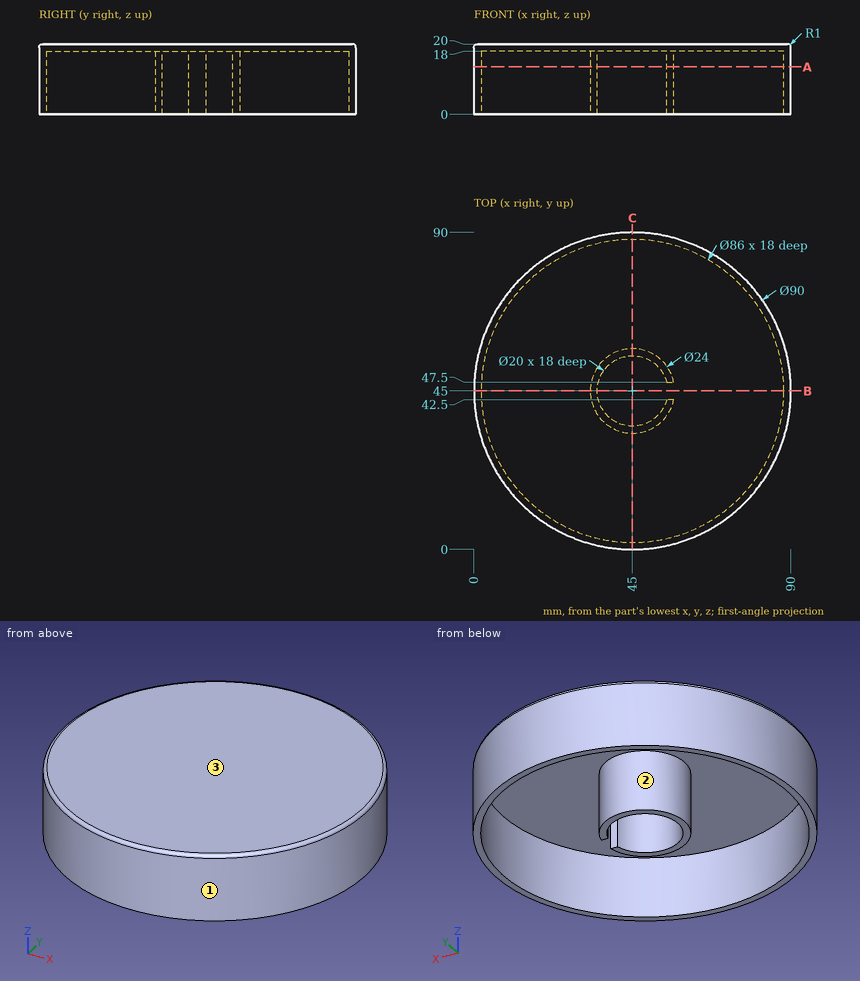
Here's the drawing with two shaded views (mm, measured from the low corner). I have some questions. Coordinates: 2 decimals unless noted, no trailing zeros. Loops run counter-clockwise (first coordinate to the right, second up) from the corner with the lowest first, then second, coordinate; pieces in that order, holes last. Notation, with made-up numbers: M 17,48 L 38,48 A15 ccw 38,58 Z; hole C 7,36.25 d5. An arc over 180 degrees is marked long. Return JSON: item names as keys, results as strings. Group by question number.
Item 1: I'm going to push flat-ended pins straight in: pin 1 Ø5 at (x, z) = (30, 8.5) entering from +Y; pin 2 Ø2.5 at (x, z) = (56, 4.5) entering from +Y; pin 3 Ø0.6 at (x, z) = (55.5, 5) entering from -Y. Where does each tip first touch, or does it pass through?
Item 2: Thinking about a two-plate mould opening in X: for the marked faces 1, 2 and 3, which applies, released by +X, released by -X, zero draft, split by the parting line, or undercut?
Item 3: Imagine slicing it at B-B (y = 45). Please give me the cut outline in (x, z), and give its area (3 significant figures).
Item 4: If I drill on L1, parallel to Y at x = 45, z = 12.75; L2, parallel to X at y = 45.5, z = 17.25; L3, parallel to X at y = 50.5, z = 6.5, over which ranges is the centre line in solid material (lowest first)? Write a range as from..to.
Item 5: Imagine slicing it at A-A (z = 13.5). Please give me the cut outline in (x, y), and give its area (3 significant figures).
Item 6: Imagine slicing it at C-C (x = 45). Please give me the cut outline in (y, z), and give its area (3 significant figures).
Verdict:
{
 "1": {"pin 1": "stops at y = 88.23", "pin 2": "stops at y = 88.93", "pin 3": "stops at y = 1.17"},
 "2": {"face 1": "split by the parting line", "face 2": "undercut", "face 3": "zero draft"},
 "3": {"outline": "M 0,0 L 2,0 L 2,18 L 33,18 L 33,0 L 35,0 L 35,18 L 88,18 L 88,0 L 90,0 L 90,19 A1 ccw 89,20 L 1,20 A1 ccw 0,19 Z", "area": "288 mm^2"},
 "4": {"L1": "y = 0..2, 33..35, 55..57, 88..90", "L2": "x = 0..2, 33.01..35.01, 88..90", "L3": "x = 0.34..2.35, 34.33..36.65, 53.35..55.67, 87.65..89.66"},
 "5": {"outline": "C 45,45 d90; M 54.68,42.5 A10 cw long 54.68,47.5 L 56.74,47.5 A12 ccw long 56.74,42.5 Z; hole C 45,45 d86", "area": "681 mm^2"},
 "6": {"outline": "M 0,0 L 2,0 L 2,18 L 33,18 L 33,0 L 35,0 L 35,18 L 55,18 L 55,0 L 57,0 L 57,18 L 88,18 L 88,0 L 90,0 L 90,19 A1 ccw 89,20 L 1,20 A1 ccw 0,19 Z", "area": "324 mm^2"}
}
